```python
from build123d import *

# Parameters (mm, degrees)
BOSS_EXTRUDE1_DEPTH = 1
SKETCH2_R           = 1.5
SKETCH2_R_2         = 2.5
CUT_EXTRUDE2_DEPTH  = 1
SKETCH3_R           = 1.5
CUT_EXTRUDE3_DEPTH  = 1


with BuildPart() as part:
    # Sketch1 → Boss-Extrude1 (new body)
    with BuildSketch(Plane(origin=(0, 0, 0), x_dir=(1, 0, 0), z_dir=(0, 1, 0))):
        with BuildLine():
            Line((2, 0), (98, 0))
            ThreePointArc((98, 0), (99.414213562, 0.585786438), (100, 2))
            Line((100, 2), (100, 98))
            ThreePointArc((100, 98), (99.414213562, 99.414213562), (98, 100))
            Line((98, 100), (2, 100))
            ThreePointArc((2, 100), (0.585786438, 99.414213562), (0, 98))
            Line((0, 98), (0, 2))
            ThreePointArc((0, 2), (0.585786438, 0.585786438), (2, 0))
        make_face()
        with BuildLine():
            Line((10, 21.5), (90, 21.5))
            ThreePointArc((90, 21.5), (91.5, 20), (90, 18.5))
            Line((90, 18.5), (10, 18.5))
            ThreePointArc((10, 18.5), (8.5, 20), (10, 21.5))
        make_face(mode=Mode.SUBTRACT)
    extrude(amount=BOSS_EXTRUDE1_DEPTH)

    # Sketch2 → Cut-Extrude2 (cut)
    with BuildSketch(Plane(origin=(0, 1, 0), x_dir=(1, 0, 0), z_dir=(0, 1, 0))):
        with BuildLine():
            Line((0, 100), (0, 65))
            Line((0, 65), (19, 65))
            ThreePointArc((19, 65), (19.707106781, 65.292893219), (20, 66))
            Line((20, 66), (20, 100))
            Line((20, 100), (0, 100))
        make_face()
        with BuildLine():
            Line((100, 65), (100, 100))
            Line((100, 100), (80, 100))
            Line((80, 100), (80, 66))
            ThreePointArc((80, 66), (80.292893219, 65.292893219), (81, 65))
            Line((81, 65), (100, 65))
        make_face()
        with Locations(Location((26, 91.5, 0), (0, 0, 270))):
            Circle(SKETCH2_R)
        with Locations(Location((26, 73.5, 0), (0, 0, 90))):
            Circle(SKETCH2_R)
        with Locations(Location((74, 91.5, 0), (0, 0, 270))):
            Circle(SKETCH2_R)
        with Locations(Location((74, 73.5, 0), (0, 0, 270))):
            Circle(SKETCH2_R)
        with Locations(Location((15, 26.5, 0), (0, 0, 270))):
            Circle(SKETCH2_R_2)
        with Locations(Location((25, 26.5, 0), (0, 0, 270))):
            Circle(SKETCH2_R_2)
        with Locations(Location((85, 26.5, 0), (0, 0, 270))):
            Circle(SKETCH2_R_2)
        with Locations(Location((75, 26.5, 0), (0, 0, 90))):
            Circle(SKETCH2_R_2)
    extrude(amount=-CUT_EXTRUDE2_DEPTH, mode=Mode.SUBTRACT)

    # Sketch3 → Cut-Extrude3 (cut)
    with BuildSketch(Plane(origin=(0, 1, 0), x_dir=(1, 0, 0), z_dir=(0, 1, 0))):
        with Locations(Location((6, 26, 0), (0, 0, 270))):
            Circle(SKETCH3_R)
        with Locations(Location((23, 95, 0), (0, 0, 270))):
            Circle(SKETCH3_R)
        with Locations(Location((77, 95, 0), (0, 0, 270))):
            Circle(SKETCH3_R)
        with Locations(Location((94, 26, 0), (0, 0, 270))):
            Circle(SKETCH3_R)
        with Locations(Location((6, 62, 0), (0, 0, 270))):
            Circle(SKETCH3_R)
        with Locations(Location((94, 62, 0), (0, 0, 270))):
            Circle(SKETCH3_R)
    extrude(amount=-CUT_EXTRUDE3_DEPTH, mode=Mode.SUBTRACT)


solid = part.part
```
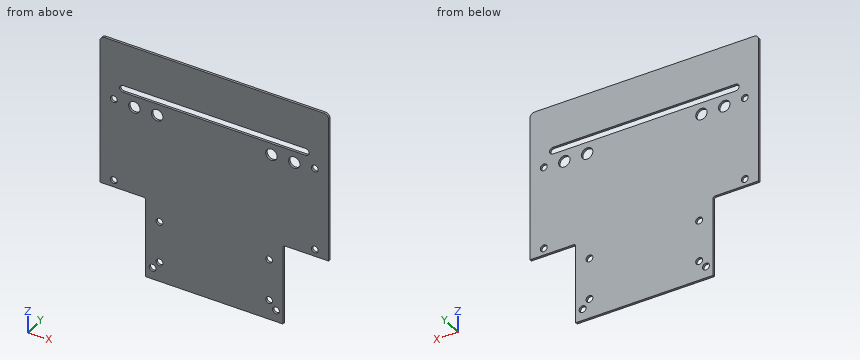
Check sheet for the modelled part. Datum: model origin and axes. Units: mm. Give positions to 0.01 mm unless a question says otherwise; leave off trailing zeros. Write each loop counter-clockwise with the first axis right and the second up, starting at its lowest first coordinate (ties: lowest second). Pieces come first, ordered by that corner, then holes.
Item 1: Cross-section at C-C (x = 94). Enter the section's corners in (y, z), and give its area (3 significant figures).
Item 2: Cross-section at B-B (y = 0.2). Count the separate pieces of the cut face and the enclosed holes in it, and give its area (3 significant figures).
Item 3: Scan lines: L1, parallel to X at y = 0.3, z = -62; L2, parallel to X at y = 0.7, z = -73.5; L3, parallel to Z at x = 88, y = 0.4. Record each from-to range of solid material in increasing order.
Item 4: Cross-section at D-D (x = 44). Enter the section's corners in (y, z).
Item 5: Cross-section at A-A (z = -73.5). Enter the section's corners in (x, y), and give its area (3 significant figures).
Report:
1. outline: (0, -65) - (1, -65) - (1, -63.5) - (0, -63.5) - close; (0, -60.5) - (1, -60.5) - (1, -27.5) - (0, -27.5) - close; (0, -24.5) - (1, -24.5) - (1, 0) - (0, 0) - close
1. area: 59.0 mm2
2. separate pieces: 1
2. enclosed holes: 15
2. area: 8,200 mm2
3. L1: x = 0 to 4.5, 7.5 to 92.5, 95.5 to 100
3. L2: x = 20 to 24.5, 27.5 to 72.5, 75.5 to 80
3. L3: z = -65 to -21.5, -18.5 to 0
4. outline: (0, -100) - (1, -100) - (1, -21.5) - (0, -21.5) - close; (0, -18.5) - (1, -18.5) - (1, 0) - (0, 0) - close
5. outline: (20, 0) - (24.5, 0) - (24.5, 1) - (20, 1) - close; (27.5, 0) - (72.5, 0) - (72.5, 1) - (27.5, 1) - close; (75.5, 0) - (80, 0) - (80, 1) - (75.5, 1) - close
5. area: 54.0 mm2
